Could you check a few things on this model? Use its own coordinates, in mm. Round coordinates to 2 decimals unless told otherwise and drop trailing zeros. Loops run counter-clockwise (first coordinate to the right, second up) from the corner with the lowest first, then second, coordinate; pieces in that order, holes last.
from build123d import *

# Parameters (mm, degrees)
BOSS_EXTRUDE1_DEPTH                                = 5.08
CSK_FOR_10_FLAT_HEAD_MACHINE_SCREW_100_D           = 2.8702
CSK_FOR_10_FLAT_HEAD_MACHINE_SCREW_100_CSINK_D     = 5.08
CSK_FOR_10_FLAT_HEAD_MACHINE_SCREW_100_CSINK_ANGLE = 82


with BuildPart() as part:
    # Sketch2 → Boss-Extrude1 (new body)
    with BuildSketch(Plane.XY):
        with BuildLine():
            Line((2.973598589, 18.816487755), (2.973598589, 9.048941177))
            ThreePointArc((2.973598589, 9.048941177), (-9.525, 0), (2.973598589, -9.048941177))
            Line((2.973598589, -9.048941177), (2.973598589, -18.816487755))
            ThreePointArc((2.973598589, -18.816487755), (-19.05, 0), (2.973598589, 18.816487755))
        make_face()
    extrude(amount=BOSS_EXTRUDE1_DEPTH)

    # CSK for #10 Flat Head Machine Screw (100)1 (through all)
    with Locations(Plane(origin=(-11.1125, 6.35, 5.08), x_dir=(1, 0, 0), z_dir=(0, 0, 1))):
        with Locations((0, 0), (0, -12.7)):
            CounterSinkHole(CSK_FOR_10_FLAT_HEAD_MACHINE_SCREW_100_D / 2, CSK_FOR_10_FLAT_HEAD_MACHINE_SCREW_100_CSINK_D / 2, counter_sink_angle=CSK_FOR_10_FLAT_HEAD_MACHINE_SCREW_100_CSINK_ANGLE)


solid = part.part
Item 1: We'd pull the mould along X, two halves only. Please class faces 1 (the cylindrical face through (-9.97, 5.48, 1.88)), 2 (the flat face through (-10, 0, 5.08)), 3 (the flat face through (2.974, 14, 3)), 4 (the cylindrical face through (-9.97, -7.22, 1.88)): released by +X, released by -X, zero draft, split by the parting line, or undercut.
Results list:
face 1: undercut
face 2: zero draft
face 3: released by +X
face 4: undercut
Item 2: If I drill on line 1 along Y through (x, z) = (-10.25, 3.85); line 2 along Y through (x, z) = (0.25, 0.5); line 3 along Y through (x, z) = (-10.5, 4.85), over which ranges is the centre line in solid material (lowest first)?
Results list:
line 1: y = -16.06 to -7.54, -5.16 to 5.16, 7.54 to 16.06
line 2: y = -19.05 to -9.52, 9.52 to 19.05
line 3: y = -15.9 to -8.61, -4.09 to 4.09, 8.61 to 15.9
Item 3: If we section it at A-A, the plane z = 1.05: Count the separate pieces of the cut face and the enclosed holes in it, then the cut area to 3 significant figures.
Results list:
separate pieces: 1
enclosed holes: 2
area: 472 mm2
Item 4: Will these pins go through, and if not, where does the flat tip stop? pin 1 (3 mm diameter, centred on x = -12.5, z = 2, fed in from -Y); pin 2 (4.5 mm diameter, centred on x = -11.11, y = 6.35, fed in from +Z); pin 3 (1.5 mm diameter, centred on y = 7.5, z = 3, fed in from -X).
Results list:
pin 1: stops at y = -15.55
pin 2: stops at z = 4.75
pin 3: stops at x = -17.81
Item 5: If we section it at D-D, the plane x = -6.5: Please give me the cut outline in (y, z).
Results list:
outline: (-17.91, 0) - (-6.96, 0) - (-6.96, 5.08) - (-17.91, 5.08) - close; (6.96, 0) - (17.91, 0) - (17.91, 5.08) - (6.96, 5.08) - close
Item 6: If we section it at C-C, the plane y = -6.35: Please give me the cut outline in (x, z).
Results list:
outline: (-17.96, 0) - (-12.55, 0) - (-12.55, 3.81) - (-13.65, 5.08) - (-17.96, 5.08) - close; (-9.68, 0) - (-7.1, 0) - (-7.1, 5.08) - (-8.57, 5.08) - (-9.68, 3.81) - close
Item 7: If we section it at B-B, the plane x = 0: Please give me the cut outline in (y, z) (3 decimals), then the cut area to 3 significant figures.
Results list:
outline: (-19.05, 0) - (-9.525, 0) - (-9.525, 5.08) - (-19.05, 5.08) - close; (9.525, 0) - (19.05, 0) - (19.05, 5.08) - (9.525, 5.08) - close
area: 96.8 mm2
